```python
from build123d import *

# Parameters (mm, degrees)
F1_DEPTH     = 50.8
F2_DEPTH     = 12.7
F4_D         = 17.272
F5_DEPTH     = 76.2
F6_DEPTH     = 76.2
F7_W         = 20.4321481287
F7_H         = 32.4622914195
F8_DEPTH     = 25.4
F9_R         = 7.62
F10_SIZE     = 10.16
F12_D        = 9.4234
F13_DEPTH    = 12.7
F14_T1_DEPTH = 101.6


# Not quite as in the source:
# - a fillet or chamfer that OpenCascade refuses, or shapes differently, is made with other operations: its cross-section is extruded or revolved along the edge and cut away or added


with BuildPart() as f1:
    # F0 (on Top) → F1 (new body, symmetric)
    with BuildSketch(Plane.XY):
        Polygon((-44.3969555199, 12.5075299293), (-44.3969555199, 14.226121828), (-55.4723292589, 14.226121828), (-55.4723292589, -39.2411798239), (53.3718280494, -39.2411798239), (53.3718280494, 14.226121828), (39.0502288938, 14.226121828), (39.0502288938, 10.7889380306), (6.9698439911, 10.7889380306), (6.9698439911, 14.226121828), (-13.0803938955, 14.226121828), (-13.0803938955, 12.5075299293), align=None)
    extrude(amount=F1_DEPTH, both=True)

    # F2 (add): a face of the model
    f2_faces = [f1.faces().sort_by_distance(p)[0] for p in [
        (-3.0552749522, 14.226121828, 0),
    ]]
    extrude(f2_faces, amount=F2_DEPTH)

    # F4 (through all)
    with Locations(Plane(origin=(0, 0, -50.8), x_dir=(1, 0, 0), z_dir=(0, 0, -1))):
        with Locations((-1.0502506047, 12.507528998)):
            Hole(F4_D / 2)

    # F5 (add): a face of the model
    f5_faces = [f1.faces().sort_by_distance(p)[0] for p in [
        (-45.6707358145, 13.3668258786, 50.8),
    ]]
    extrude(f5_faces, amount=-F5_DEPTH)

    # F6 (add): a face of the model
    f6_faces = [f1.faces().sort_by_distance(p)[0] for p in [
        (-45.6707358145, 13.3668258786, 50.8),
    ]]
    extrude(f6_faces, amount=-F6_DEPTH)

    # F7 (on face) → F8 (join)
    with BuildSketch(Plane.YZ.offset(53.3718280494)):
        with Locations((-15.8492363989, -0.2864319831)):
            Rectangle(F7_W, F7_H)
    extrude(amount=F8_DEPTH)

    # F9
    f9_edges = [f1.edges().sort_by_distance(p)[0] for p in [
        (-13.080394, 26.926122, 0),
        (6.969844, 26.926122, 0),
    ]]
    fillet(f9_edges, radius=F9_R)

    # F10
    f10_edges = [f1.edges().sort_by_distance(p)[0] for p in [
        (53.371828, -39.24118, 0),
        (-55.472329, -39.24118, 0),
    ]]
    chamfer(f10_edges, length=F10_SIZE)

    # F12 (through all)
    with Locations(Plane.YZ.offset(78.7718280494)):
        with Locations((-15.8492363989, -0.2864319831)):
            Hole(F12_D / 2)

    # F13 (add): a face of the model
    f13_faces = [f1.faces().sort_by_distance(p)[0] for p in [
        (-3.0552749522, 26.926121828, 0),
    ]]
    extrude(f13_faces, amount=F13_DEPTH)

    # F14: fillet of radius 5.08 on 2 edges, made by hand

    # F14_s2 → F14_t1 (join)
    with BuildSketch(Plane.XY.offset(-50.8)):
        with BuildLine():
            ThreePointArc((-44.3969555199, 14.226121828), (-42.6774175907, 12.9570681189), (-40.5881058804, 12.5075299293))
            Line((-40.5881058804, 12.5075299293), (-44.3969555199, 12.5075299293))
            Line((-44.3969555199, 12.5075299293), (-44.3969555199, 14.226121828))
        make_face()
        with BuildLine():
            ThreePointArc((39.0502288938, 14.226121828), (37.1979300298, 11.7366319971), (34.2431970731, 10.7889380306))
            Line((34.2431970731, 10.7889380306), (39.0502288938, 10.7889380306))
            Line((39.0502288938, 10.7889380306), (39.0502288938, 14.226121828))
        make_face()
    extrude(amount=F14_T1_DEPTH)


solid = f1.part
```
Input: part model. Units: mm. Frame: model coordinates. A direction names the side the tool comes from. Give positions to 0.01 mm unless a question says otherwise; leave off trailing zeros. Order: outer loops, then holes, each group sorted by start corner. A loop starts at its lowest first (then second) coordinate and runs counter-clockwise, first axis right, second up. Notation, with made-up numbers: M -33.75,62.5 L 20.25,62.5 A21 cw 20.25,82.5 Z; hole C -30.5,66 d7. An arc over 180 degrees is marked long. Return JSON: item names as keys, results as strings.
Item 1: Cut plane B-B (x = -22). Return loops of the section in (y, z), then the cut area to 3 significant figures.
Solutions:
{"outline": "M -39.24,-50.8 L 12.51,-50.8 L 12.51,50.8 L -39.24,50.8 Z; hole C -15.85,-0.29 d9.42", "area": "5,190 mm^2"}
Item 2: First-contact query: P1, Ø3, axis at y = 30, z = 31.5, coming from the -X side; P2, Ø9, axis at x = -51, z = 1, coming from the +Y side; P3, Ø8.5, axis at x = -27.5, z = -5.5, coming from the +Y side. Flat tips, straight axial feed; report the tip coordinate or a pass-through.
Solutions:
{"P1": "x = -5.46", "P2": "y = 14.23", "P3": "y = 12.51"}
Item 3: Cut plane A-A (z = 10). Return loops of the section in (x, y), then the cut area to 3 significant figures.
Solutions:
{"outline": "M -55.47,-29.08 L -45.31,-39.24 L 43.21,-39.24 L 53.37,-29.08 L 53.37,-26.07 L 78.77,-26.07 L 78.77,-5.63 L 53.37,-5.63 L 53.37,14.23 L 39.05,14.23 A5.08 cw 34.24,10.79 L 6.97,10.79 L 6.97,19.31 A7.62 ccw -0.65,26.93 L -0.65,39.63 L -5.46,39.63 L -5.46,26.93 A7.62 ccw -13.08,19.31 L -13.08,12.51 L -40.59,12.51 A5.08 cw -44.4,14.23 L -55.47,14.23 Z; hole C -1.05,-12.51 d17.27", "area": "6,130 mm^2"}
Item 4: Pull-direction query (X, two-part tool) for faces 1 (the cylindrical face through (0.822, -4.077, 0.711)), 2 (the flat face through (-3, 39.626, 1)), 3 (the cylindrical face through (37.23, 11.76, -0.71)), 4 (the flat face through (-5.46, 33, -1)); classes: +X half, -X half, draft (parallel to the pull), parting line (faces both ways), or undercut.
Solutions:
{"face 1": "undercut", "face 2": "draft", "face 3": "undercut", "face 4": "-X half"}
Item 5: Cut plane C-C (y = 16.5). Return loops of the section in (x, z).
Solutions:
{"outline": "M -13.08,-50.8 L 6.97,-50.8 L 6.97,50.8 L -13.08,50.8 Z"}
Item 6: Ray query, probe 1 along X at (y, z) = (-12, -45); probe 2 along X at (y, z) = (13.5, 34); probe 3 along Y at (x, z) = (-1, -20). Return the intervals inside material, ascending.
Solutions:
{"probe 1": "-55.47 to -9.67, 7.57 to 53.37", "probe 2": "-55.47 to -43.6, -13.08 to 6.97, 38.74 to 53.37", "probe 3": "-39.24 to -21.14, -3.87 to 39.63"}
Item 7: Access query for faces 5 (the flat face through (66, -16, 15.945)), 6 (the flat face through (-27, 12.508, 1)), 7 (the flat face through (66, -26.065, -1)), 8 (the flat face through (46, 14.226, 1)). Directions: +Z, -Z, +X, -X, +Y, -Y. A direction counts if a zero-diameter tool reaches every point of the face in a straight line with its end or side. Return the directions, or none.
Solutions:
{"face 5": "+Z, +X, +Y, -Y", "face 6": "+Z, -Z, +Y", "face 7": "+Z, -Z, +X, -Y", "face 8": "+Z, -Z, +X, +Y"}
Item 8: Cut plane D-D (z = 33). Return loops of the section in (x, y), then the cut area to 3 significant figures.
Solutions:
{"outline": "M -55.47,-29.08 L -45.31,-39.24 L 43.21,-39.24 L 53.37,-29.08 L 53.37,14.23 L 39.05,14.23 A5.08 cw 34.24,10.79 L 6.97,10.79 L 6.97,19.31 A7.62 ccw -0.65,26.93 L -0.65,39.63 L -5.46,39.63 L -5.46,26.93 A7.62 ccw -13.08,19.31 L -13.08,12.51 L -40.59,12.51 A5.08 cw -44.4,14.23 L -55.47,14.23 Z; hole C -1.05,-12.51 d17.27", "area": "5,620 mm^2"}
